Read the model definition and answer for the solid it produces. Units are mm, in the model's axes. A direction names the side the tool comes from. Coordinates: 2 decimals unless noted, no trailing zeros. Loops run counter-clockwise (first coordinate to the right, second up) from the corner with the lowest first, then second, coordinate; pieces in that order, holes last. Notation, with made-up numbers: (-21, 14.25) -> (19, 14.25) arc R31 ccw to (19, 41.25) -> close; hole circle Ø3 at (-11, -39.5). An arc over 180 degrees is marked (long way). Answer in a Markdown table with one row per item.
```python
from build123d import *

# Parameters (mm, degrees)
FRONT_GRIP_ACETAL_GUIDE_COMB_SKETCH_W  = 6
FRONT_GRIP_ACETAL_GUIDE_COMB_SKETCH_H  = 53
FRONT_GRIP_ACETAL_GUIDE_COMB_DEPTH     = 2.5
GRIP_GUIDE_LEDGE_1_LOWER_SKETCH_W      = 32.1
GRIP_GUIDE_LEDGE_1_LOWER_SKETCH_H      = 4.1
GRIP_GUIDE_LEDGE_1_LOWER_DEPTH         = 2.5
GRIP_GUIDE_LEDGE_1_UPPER_SKETCH_W      = 32.1
GRIP_GUIDE_LEDGE_1_UPPER_SKETCH_H      = 4.1
GRIP_GUIDE_LEDGE_1_UPPER_DEPTH         = 2.5
GRIP_GUIDE_FENCE_1_LOWER_SKETCH_W      = 24
GRIP_GUIDE_FENCE_1_LOWER_SKETCH_H      = 1.1
GRIP_GUIDE_FENCE_1_LOWER_DEPTH         = 1.5
GRIP_GUIDE_FENCE_1_UPPER_SKETCH_W      = 24
GRIP_GUIDE_FENCE_1_UPPER_SKETCH_H      = 1.1
GRIP_GUIDE_FENCE_1_UPPER_DEPTH         = 1.5
GRIP_GUIDE_LEDGE_2_LOWER_SKETCH_W      = 32.1
GRIP_GUIDE_LEDGE_2_LOWER_SKETCH_H      = 4.1
GRIP_GUIDE_LEDGE_2_LOWER_DEPTH         = 2.5
GRIP_GUIDE_LEDGE_2_UPPER_SKETCH_W      = 32.1
GRIP_GUIDE_LEDGE_2_UPPER_SKETCH_H      = 4.1
GRIP_GUIDE_LEDGE_2_UPPER_DEPTH         = 2.5
GRIP_GUIDE_FENCE_2_LOWER_SKETCH_W      = 24
GRIP_GUIDE_FENCE_2_LOWER_SKETCH_H      = 1.1
GRIP_GUIDE_FENCE_2_LOWER_DEPTH         = 1.5
GRIP_GUIDE_FENCE_2_UPPER_SKETCH_W      = 24
GRIP_GUIDE_FENCE_2_UPPER_SKETCH_H      = 1.1
GRIP_GUIDE_FENCE_2_UPPER_DEPTH         = 1.5
GRIP_GUIDE_LEDGE_3_LOWER_SKETCH_W      = 32.1
GRIP_GUIDE_LEDGE_3_LOWER_SKETCH_H      = 4.1
GRIP_GUIDE_LEDGE_3_LOWER_DEPTH         = 2.5
GRIP_GUIDE_LEDGE_3_UPPER_SKETCH_W      = 32.1
GRIP_GUIDE_LEDGE_3_UPPER_SKETCH_H      = 4.1
GRIP_GUIDE_LEDGE_3_UPPER_DEPTH         = 2.5
GRIP_GUIDE_FENCE_3_LOWER_SKETCH_W      = 24
GRIP_GUIDE_FENCE_3_LOWER_SKETCH_H      = 1.1
GRIP_GUIDE_FENCE_3_LOWER_DEPTH         = 1.5
GRIP_GUIDE_FENCE_3_UPPER_SKETCH_W      = 24
GRIP_GUIDE_FENCE_3_UPPER_SKETCH_H      = 1.1
GRIP_GUIDE_FENCE_3_UPPER_DEPTH         = 1.5
FRONT_GUIDE_SCREW_CLEARANCE_1_SKETCH_R = 1.1
FRONT_GUIDE_SCREW_CLEARANCE_1_DEPTH    = 2.7
FRONT_GUIDE_SCREW_CLEARANCE_2_SKETCH_R = 1.1
FRONT_GUIDE_SCREW_CLEARANCE_2_DEPTH    = 2.7
OUTLET_SEAT_CLEARANCE_1_SKETCH_R       = 4.75
OUTLET_SEAT_CLEARANCE_1_DEPTH          = 2.2
OUTLET_SEAT_CLEARANCE_2_SKETCH_R       = 4.75
OUTLET_SEAT_CLEARANCE_2_DEPTH          = 2.2
OUTLET_SEAT_CLEARANCE_3_SKETCH_R       = 4.75
OUTLET_SEAT_CLEARANCE_3_DEPTH          = 2.2


with BuildPart() as part:
    # Front Grip Acetal Guide Comb sketch → Front Grip Acetal Guide Comb (new body)
    with BuildSketch(Plane.XY.offset(8.5)):
        with Locations((-63.291651246, -29)):
            Rectangle(FRONT_GRIP_ACETAL_GUIDE_COMB_SKETCH_W, FRONT_GRIP_ACETAL_GUIDE_COMB_SKETCH_H)
    extrude(amount=FRONT_GRIP_ACETAL_GUIDE_COMB_DEPTH)

    # Grip Guide Ledge 1 Lower sketch → Grip Guide Ledge 1 Lower (add)
    with BuildSketch(Plane.XY.offset(8.5)):
        with Locations((-44.341651246, -6.75)):
            Rectangle(GRIP_GUIDE_LEDGE_1_LOWER_SKETCH_W, GRIP_GUIDE_LEDGE_1_LOWER_SKETCH_H)
    extrude(amount=GRIP_GUIDE_LEDGE_1_LOWER_DEPTH)

    # Grip Guide Ledge 1 Upper sketch → Grip Guide Ledge 1 Upper (add)
    with BuildSketch(Plane.XY.offset(8.5)):
        with Locations((-44.341651246, -17.25)):
            Rectangle(GRIP_GUIDE_LEDGE_1_UPPER_SKETCH_W, GRIP_GUIDE_LEDGE_1_UPPER_SKETCH_H)
    extrude(amount=GRIP_GUIDE_LEDGE_1_UPPER_DEPTH)

    # Grip Guide Fence 1 Lower sketch → Grip Guide Fence 1 Lower (add)
    with BuildSketch(Plane.XY.offset(10.9)):
        with Locations((-40.291651246, -5.25)):
            Rectangle(GRIP_GUIDE_FENCE_1_LOWER_SKETCH_W, GRIP_GUIDE_FENCE_1_LOWER_SKETCH_H)
    extrude(amount=GRIP_GUIDE_FENCE_1_LOWER_DEPTH)

    # Grip Guide Fence 1 Upper sketch → Grip Guide Fence 1 Upper (add)
    with BuildSketch(Plane.XY.offset(10.9)):
        with Locations((-40.291651246, -18.75)):
            Rectangle(GRIP_GUIDE_FENCE_1_UPPER_SKETCH_W, GRIP_GUIDE_FENCE_1_UPPER_SKETCH_H)
    extrude(amount=GRIP_GUIDE_FENCE_1_UPPER_DEPTH)

    # Grip Guide Ledge 2 Lower sketch → Grip Guide Ledge 2 Lower (add)
    with BuildSketch(Plane.XY.offset(8.5)):
        with Locations((-44.341651246, -23.75)):
            Rectangle(GRIP_GUIDE_LEDGE_2_LOWER_SKETCH_W, GRIP_GUIDE_LEDGE_2_LOWER_SKETCH_H)
    extrude(amount=GRIP_GUIDE_LEDGE_2_LOWER_DEPTH)

    # Grip Guide Ledge 2 Upper sketch → Grip Guide Ledge 2 Upper (add)
    with BuildSketch(Plane.XY.offset(8.5)):
        with Locations((-44.341651246, -34.25)):
            Rectangle(GRIP_GUIDE_LEDGE_2_UPPER_SKETCH_W, GRIP_GUIDE_LEDGE_2_UPPER_SKETCH_H)
    extrude(amount=GRIP_GUIDE_LEDGE_2_UPPER_DEPTH)

    # Grip Guide Fence 2 Lower sketch → Grip Guide Fence 2 Lower (add)
    with BuildSketch(Plane.XY.offset(10.9)):
        with Locations((-40.291651246, -22.25)):
            Rectangle(GRIP_GUIDE_FENCE_2_LOWER_SKETCH_W, GRIP_GUIDE_FENCE_2_LOWER_SKETCH_H)
    extrude(amount=GRIP_GUIDE_FENCE_2_LOWER_DEPTH)

    # Grip Guide Fence 2 Upper sketch → Grip Guide Fence 2 Upper (add)
    with BuildSketch(Plane.XY.offset(10.9)):
        with Locations((-40.291651246, -35.75)):
            Rectangle(GRIP_GUIDE_FENCE_2_UPPER_SKETCH_W, GRIP_GUIDE_FENCE_2_UPPER_SKETCH_H)
    extrude(amount=GRIP_GUIDE_FENCE_2_UPPER_DEPTH)

    # Grip Guide Ledge 3 Lower sketch → Grip Guide Ledge 3 Lower (add)
    with BuildSketch(Plane.XY.offset(8.5)):
        with Locations((-44.341651246, -40.75)):
            Rectangle(GRIP_GUIDE_LEDGE_3_LOWER_SKETCH_W, GRIP_GUIDE_LEDGE_3_LOWER_SKETCH_H)
    extrude(amount=GRIP_GUIDE_LEDGE_3_LOWER_DEPTH)

    # Grip Guide Ledge 3 Upper sketch → Grip Guide Ledge 3 Upper (add)
    with BuildSketch(Plane.XY.offset(8.5)):
        with Locations((-44.341651246, -51.25)):
            Rectangle(GRIP_GUIDE_LEDGE_3_UPPER_SKETCH_W, GRIP_GUIDE_LEDGE_3_UPPER_SKETCH_H)
    extrude(amount=GRIP_GUIDE_LEDGE_3_UPPER_DEPTH)

    # Grip Guide Fence 3 Lower sketch → Grip Guide Fence 3 Lower (add)
    with BuildSketch(Plane.XY.offset(10.9)):
        with Locations((-40.291651246, -39.25)):
            Rectangle(GRIP_GUIDE_FENCE_3_LOWER_SKETCH_W, GRIP_GUIDE_FENCE_3_LOWER_SKETCH_H)
    extrude(amount=GRIP_GUIDE_FENCE_3_LOWER_DEPTH)

    # Grip Guide Fence 3 Upper sketch → Grip Guide Fence 3 Upper (add)
    with BuildSketch(Plane.XY.offset(10.9)):
        with Locations((-40.291651246, -52.75)):
            Rectangle(GRIP_GUIDE_FENCE_3_UPPER_SKETCH_W, GRIP_GUIDE_FENCE_3_UPPER_SKETCH_H)
    extrude(amount=GRIP_GUIDE_FENCE_3_UPPER_DEPTH)

    # Front Guide Screw Clearance 1 sketch → Front Guide Screw Clearance 1 (cut)
    with BuildSketch(Plane.XY.offset(8.4)):
        with Locations(Location((-63.291651246, -5.5, 0), (0, 0, 180))):
            Circle(FRONT_GUIDE_SCREW_CLEARANCE_1_SKETCH_R)
    extrude(amount=FRONT_GUIDE_SCREW_CLEARANCE_1_DEPTH, mode=Mode.SUBTRACT)

    # Front Guide Screw Clearance 2 sketch → Front Guide Screw Clearance 2 (cut)
    with BuildSketch(Plane.XY.offset(8.4)):
        with Locations(Location((-63.291651246, -52.5, 0), (0, 0, 180))):
            Circle(FRONT_GUIDE_SCREW_CLEARANCE_2_SKETCH_R)
    extrude(amount=FRONT_GUIDE_SCREW_CLEARANCE_2_DEPTH, mode=Mode.SUBTRACT)

    # Outlet seat clearance 1 sketch → Outlet seat clearance 1 (cut)
    with BuildSketch(Plane(origin=(-62.391651246, 0, 0), x_dir=(0, 0, -1), z_dir=(1, 0, 0))):
        with Locations((-15, -12)):
            Circle(OUTLET_SEAT_CLEARANCE_1_SKETCH_R)
    extrude(amount=OUTLET_SEAT_CLEARANCE_1_DEPTH, mode=Mode.SUBTRACT)

    # Outlet seat clearance 2 sketch → Outlet seat clearance 2 (cut)
    with BuildSketch(Plane(origin=(-62.391651246, 0, 0), x_dir=(0, 0, -1), z_dir=(1, 0, 0))):
        with Locations((-15, -29)):
            Circle(OUTLET_SEAT_CLEARANCE_2_SKETCH_R)
    extrude(amount=OUTLET_SEAT_CLEARANCE_2_DEPTH, mode=Mode.SUBTRACT)

    # Outlet seat clearance 3 sketch → Outlet seat clearance 3 (cut)
    with BuildSketch(Plane(origin=(-62.391651246, 0, 0), x_dir=(0, 0, -1), z_dir=(1, 0, 0))):
        with Locations((-15, -46)):
            Circle(OUTLET_SEAT_CLEARANCE_3_SKETCH_R)
    extrude(amount=OUTLET_SEAT_CLEARANCE_3_DEPTH, mode=Mode.SUBTRACT)


with BuildPart() as body_2:
    # Mirror1: mirrored copy
    add(part.part.mirror(Plane(origin=(0, 0, 0), x_dir=(0, 0, 1), z_dir=(0, -1, 0))))


solid = body_2.part
```
1. A cutting plane is placed at C-C on y = 20.5. Give the vertices of the cut face in (x, z).
A:
| item | result |
|---|---|
| outline | (-66.29, 8.5) -> (-60.29, 8.5) -> (-60.29, 11) -> (-66.29, 11) -> close |
2. Given pin 1 Ø0.5 at (y, z) = (39.5, 12) entering from -X; pin 2 Ø0.8 at (y, z) = (47, 10.5) entering from +X; pin 3 Ø1.1 at (x, z) = (-36.5, 11.5) entering from -Y, each flat-ended and moving along its own axis, determine where each tip first touches the part or whether it passes through.
A:
| item | result |
|---|---|
| pin 1 | stops at x = -52.29 |
| pin 2 | stops at x = -60.29 |
| pin 3 | stops at y = 4.7 |
3. The mould has two halves that part along Y. Classify faces 1 (the flat face through (-45, 53.3, 10)), 2 (the flat face through (-45, 36.3, 10)), 3 (the flat face through (-45, 4.7, 10)), 4 (the flat face through (-28.292, 7, 10)): pulls with the +Y half, pulls with the -Y half, needs draft (parallel to the pull), parting line crosses it, or undercut.
A:
| item | result |
|---|---|
| face 1 | pulls with the +Y half |
| face 2 | undercut |
| face 3 | pulls with the -Y half |
| face 4 | needs draft |
4. A cutting plane is placed at A-A on z = 9.4. Count the separate pieces of the cut face and the enclosed holes in it, and give its area (3 significant figures).
A:
| item | result |
|---|---|
| separate pieces | 1 |
| enclosed holes | 2 |
| area | 1,100 mm2 |
5. Find the intervals of material crossed by probe 1 along Y at (x, z) = (-59.5, 9.8); probe 2 along Y at (x, z) = (-45.5, 11.4); probe 3 along X at (y, z) = (5.5, 9.25), in increasing order.
A:
| item | result |
|---|---|
| probe 1 | y = 4.7 to 8.8, 15.2 to 19.3, 21.7 to 25.8, 32.2 to 36.3, 38.7 to 42.8, 49.2 to 53.3 |
| probe 2 | y = 4.7 to 5.8, 18.2 to 19.3, 21.7 to 22.8, 35.2 to 36.3, 38.7 to 39.8, 52.2 to 53.3 |
| probe 3 | x = -66.29 to -64.39, -62.19 to -28.29 |
6. A cutting plane is placed at D-D on y = 48. Give the vertices of the cut face in (x, z), and give its area (3 significant figures).
A:
| item | result |
|---|---|
| outline | (-66.29, 8.5) -> (-60.29, 8.5) -> (-60.29, 10.69) -> (-62.39, 10.69) -> (-62.39, 11) -> (-66.29, 11) -> close |
| area | 14.4 mm2 |
7. A tool of negligible diameter and unlimited length cuts with its end or side. For faces 5 (the flat face through (-40, 39.8, 12)), 6 (the flat face through (-45, 21.7, 10)), 7 (the cylindrical face through (-61.36, 12.04, 10.25)), from which of +Z, -Z, +X, -X, +Y, -Y can it reach the whole face along a straight path? Write none if from no direction.
A:
| item | result |
|---|---|
| face 5 | +Z, +X, -X |
| face 6 | +Z, -Z, +X |
| face 7 | +Z, +X |
